Verification items for the finished model (mm, model axes). A direction names the side the tool comes from. Round coordinates to 2 decimals unless told otherwise and drop trailing zeros. Loops run counter-clockwise (first coordinate to the right, second up) from the corner with the lowest first, then second, coordinate; pieces in that order, holes last. Notation, with made-up numbers: (11.5, 82) - (32.5, 82) arc R38 ccw to (32.5, 121) - close; hole circle Ø5 at (-20, 78). An arc over 180 degrees is marked (long way). Use a Markdown table: item, result. Add a question column.
```python
from build123d import *

# Parameters (mm, degrees)
SKETCH_1_R               = 33.5
EXTRUDE_1_DEPTH          = 23
HOLE_WIZARD_1_D          = 4.5
HOLE_WIZARD_2_D          = 9
HOLE_WIZARD_3_D          = 25
SKETCH_9_W               = 10
SKETCH_9_H               = 15
CUT_EXTRUDE_1_DEPTH      = 30
PATTERN_CIRCULAR_1_COUNT = 3
SKETCH_10_W              = 67
SKETCH_10_H              = 23
CUT_EXTRUDE_2_DEPTH      = 10


with BuildPart() as part:
    # 草图1 → 凸台-拉伸1 (new body)
    with BuildSketch(Plane(origin=(0, 0, 0), x_dir=(1, 0, 0), z_dir=(0, 1, 0))):
        with Locations(Location((0, 0, 0), (0, 0, 270))):
            Circle(SKETCH_1_R)
    extrude(amount=EXTRUDE_1_DEPTH)

    # 孔1 (through all)
    with Locations(Plane(origin=(0, 23, 0), x_dir=(1, 0, 0), z_dir=(0, 1, 0))):
        with Locations((0, 29), (-25.11473671, -14.5), (25.11473671, -14.5)):
            Hole(HOLE_WIZARD_1_D / 2)

    # 孔2 (through all)
    with Locations(Plane(origin=(0, 23, 0), x_dir=(1, 0, 0), z_dir=(0, 1, 0))):
        with Locations((0, 19.25)):
            Hole(HOLE_WIZARD_2_D / 2)

    # 孔3 (through all)
    with Locations(Plane(origin=(0, 23, 0), x_dir=(1, 0, 0), z_dir=(0, 1, 0))):
        with Locations((0, 0)):
            Hole(HOLE_WIZARD_3_D / 2)

    # 草图9 → 切除-拉伸1 (cut)
    with BuildSketch(Plane.XY.offset(33.5)):
        with Locations((5, 11.5)):
            Rectangle(SKETCH_9_W, SKETCH_9_H)
        with Locations((-5, 11.5)):
            Rectangle(SKETCH_9_W, SKETCH_9_H)
    cut_extrude_1 = extrude(amount=-CUT_EXTRUDE_1_DEPTH, mode=Mode.SUBTRACT)

    # 阵列(圆周)1: 切除-拉伸1 ×3 about axis
    pattern_circular_1_axis = Axis((0, 0, 0), (0, 1, 0))
    for i in range(1, PATTERN_CIRCULAR_1_COUNT):
        add(cut_extrude_1.rotate(pattern_circular_1_axis, i * 360 / PATTERN_CIRCULAR_1_COUNT), mode=Mode.SUBTRACT)

    # 草图10 → 切除-拉伸2 (cut)
    with BuildSketch(Plane.XY.offset(33.5)):
        with Locations((0, 11.5)):
            Rectangle(SKETCH_10_W, SKETCH_10_H)
    extrude(amount=-CUT_EXTRUDE_2_DEPTH, mode=Mode.SUBTRACT)


solid = part.part
```
Q1. Section check A-A on y = 18. Record the cut outline in (x, z).
Q2. Section check B-B on z = 0. Record the cut outline in (x, y), plus the area to 3 significant figures.
Q3. Set-up check for faces 4 (the face through (12.241, 11.395, -18.614)), 5 (the face through (-12.241, 11.395, -18.614)), 6 (the face through (-22.241, 11.395, -1.294)), 7 (the face through (0, 4, 17)), 8 (the face through (8, 23, -12)): record each of +Z, -Z, +X, -X, +Y, -Y from which the full face is reachable in a straight line by a thin tool's end or side.
Q4. Thickness scan on line 1 along Z through (x, y) = (0, 8.75); line 2 along Y through (x, z) = (17, -8); line 3 along X through (y, z) = (5.75, 14.5). Record the ranges inside material, lowest first.
Q5. Release check for a two-part mould opening along Z. For faces 1 (the face through (-20, 19, -12)), 2 (the face through (8, 0, -12)), 3 (the face through (-0.3, 19.3, 23.5)) record: +Z half, -Z half, draft (parallel to the pull), parting line (faces both ways), or undercut.
Q6. Section check C-C on x = 0. Record the cut outline in (y, z), plus the area to 4 significant figures.
Q7. Section check D-D on z = 14.5. Record the cut outline in (x, y).
Q8. Go/stop test with flat-tipped pins: pin 1 Ø4.5 at (y, z) = (8.5, 15) entering from -X; pin 2 Ø8 at (x, z) = (0, -19.25) entering from -Y; pin 3 Ø5 at (x, z) = (-25.11, 14.5) entering from -Y; pin 4 Ø12 at (y, z) = (8.5, 14) entering from +X. Record where each tip stops, or that it passes through.
Determined:
| question | item | result |
|---|---|---|
| 1 | outline | (-32.69, -7.33) - (-11.5, 4.91) arc R12.5 cw to (-10, 7.5) - (-10, 23.5) - (-23.87, 23.5) arc R33.5 ccw to start; (-22.69, -24.65) arc R33.5 ccw to (22.69, -24.65) - (1.5, -12.41) arc R12.5 cw to (-1.5, -12.41) - close; (10, 7.5) arc R12.5 cw to (11.5, 4.91) - (32.69, -7.33) arc R33.5 ccw to (23.87, 23.5) - (10, 23.5) - close; hole circle Ø4.5 at (-25.11, 14.5); hole circle Ø9 at (0, -19.25); hole circle Ø4.5 at (0, -29); hole circle Ø4.5 at (25.11, 14.5) |
| 2 | outline | (-33.5, 0) - (-12.5, 0) - (-12.5, 4) - (-20, 4) - (-20, 19) - (-12.5, 19) - (-12.5, 23) - (-33.5, 23) - close; (12.5, 0) - (33.5, 0) - (33.5, 23) - (12.5, 23) - (12.5, 19) - (20, 19) - (20, 4) - (12.5, 4) - close |
| 2 | area | 741 mm² |
| 3 | face 4 | +X |
| 3 | face 5 | -X |
| 3 | face 6 | none |
| 3 | face 7 | +Z |
| 3 | face 8 | +Z, -Z, +X, -X, +Y |
| 4 | line 1 | z = -33.5 to -31.25, -26.75 to -23.75, -14.75 to -12.5 |
| 4 | line 2 | y = 0 to 4, 19 to 23 |
| 4 | line 3 | x = -30.2 to -27.36, -22.86 to -10, 10 to 22.86, 27.36 to 30.2 |
| 5 | face 1 | undercut |
| 5 | face 2 | draft |
| 5 | face 3 | +Z half |
| 6 | outline | (0, -33.5) - (23, -33.5) - (23, -31.25) - (0, -31.25) - close; (0, -26.75) - (23, -26.75) - (23, -23.75) - (0, -23.75) - close; (0, -14.75) - (23, -14.75) - (23, -12.5) - (0, -12.5) - close; (0, 12.5) - (4, 12.5) - (4, 23.5) - (0, 23.5) - close; (19, 12.5) - (23, 12.5) - (23, 23.5) - (19, 23.5) - close |
| 6 | area | 260.5 mm² |
| 7 | outline | (-30.2, 0) - (-27.36, 0) - (-27.36, 23) - (-30.2, 23) - close; (-22.86, 0) - (22.86, 0) - (22.86, 23) - (-22.86, 23) - close; (27.36, 0) - (30.2, 0) - (30.2, 23) - (27.36, 23) - close; hole (-10, 4) - (10, 4) - (10, 19) - (-10, 19) - close |
| 8 | pin 1 | stops at x = -30.98 |
| 8 | pin 2 | passes through |
| 8 | pin 3 | stops at y = 0 |
| 8 | pin 4 | stops at x = 32.53 |
